Verification items for the finished model (mm, model axes). Give positions to 0.01 mm unless a question says otherwise; leave off trailing zeros. Write each loop counter-clockwise with the first axis right and the second up, starting at its lowest first coordinate (ties: lowest second). Pieces come first, ordered by that corner, then holes. Notation, with made-up numbers: (-8, -15.75) -> (1, -15.75) arc R8 ccw to (1, -1.75) -> close; hole circle Ø2 at (-15, 8.25). An arc over 180 degrees is marked (long way). Use one line per item in the form item = value. Start each with the question number.
(1) Scan lines: L1, parallel to Z at x = -72, y = 2.3; L2, parallel to Z at x = -30, y = 0.65; L3, parallel to X at y = 0.4, z = 14.5. Record each from-to range of solid material in increasing order.
(2) Section check A-A, the plane x = 60. Record the cut outline in (y, z).
(3) Section check B-B, the plane z = 0. State how many separate pieces and enclosed holes the cut face has, plus the area to 3 significant figures.
(4) Depth check by flat-ended pin: pin 1 Ø1.5 at (x, z) = (112.5, -12) entering from -Y; pin 2 Ø4 at (x, z) = (-30, 19.5) entering from -Y. Enter the tip coordinate at first touch or a pass-through.
from build123d import *

# Parameters (mm, degrees)
SKETCH1_W               = 400
SKETCH1_H               = 55
BOSS_EXTRUDE1_DEPTH     = 2.5
SKETCH2_R               = 2.5
CUT_EXTRUDE1_DEPTH      = 2.5
LPATTERN1_COUNT         = 10
LPATTERN1_PITCH         = 40
SKETCH3_R               = 7.5
CUT_EXTRUDE2_DEPTH      = 2.5
LPATTERN2_COUNT         = 4
LPATTERN2_PITCH         = 40
MIRROR1_COPY_1_SKETCH_R = 7.5
MIRROR1_COPY_1_DEPTH    = 2.5
MIRROR1_COPY_2_SKETCH_R = 7.5
MIRROR1_COPY_2_DEPTH    = 2.5
MIRROR1_COPY_3_SKETCH_R = 7.5
MIRROR1_COPY_3_DEPTH    = 2.5
FILLET1_R               = 0.5


with BuildPart() as part:
    # Sketch1 → Boss-Extrude1 (new body)
    with BuildSketch(Plane(origin=(0, 0, 0), x_dir=(1, 0, 0), z_dir=(0, 1, 0))):
        Rectangle(SKETCH1_W, SKETCH1_H)
    extrude(amount=BOSS_EXTRUDE1_DEPTH)

    # Sketch2 → Cut-Extrude1 (cut)
    with BuildSketch(Plane(origin=(0, 2.5, 0), x_dir=(1, 0, 0), z_dir=(0, 1, 0))):
        with Locations(Location((-190, 19.5, 0), (0, 0, 270))):
            Circle(SKETCH2_R)
        with Locations(Location((-170, 19.5, 0), (0, 0, 270))):
            Circle(SKETCH2_R)
        with Locations(Location((-190, -19.5, 0), (0, 0, 270))):
            Circle(SKETCH2_R)
        with Locations(Location((-170, -19.5, 0), (0, 0, 270))):
            Circle(SKETCH2_R)
    cut_extrude1 = extrude(amount=-CUT_EXTRUDE1_DEPTH, mode=Mode.SUBTRACT)

    # LPattern1: Cut-Extrude1 ×10
    with Locations(*[(i * LPATTERN1_PITCH, 0, 0) for i in range(1, LPATTERN1_COUNT)]):
        add(cut_extrude1, mode=Mode.SUBTRACT)

    # Sketch3 → Cut-Extrude2 (cut)
    with BuildSketch(Plane(origin=(0, 2.5, 0), x_dir=(1, 0, 0), z_dir=(0, 1, 0))):
        with Locations(Location((-180, 0, 0), (0, 0, 270))):
            Circle(SKETCH3_R)
    cut_extrude2 = extrude(amount=-CUT_EXTRUDE2_DEPTH, mode=Mode.SUBTRACT)

    # LPattern2: Cut-Extrude2 ×4
    with Locations(*[(i * LPATTERN2_PITCH, 0, 0) for i in range(1, LPATTERN2_COUNT)]):
        add(cut_extrude2, mode=Mode.SUBTRACT)

    # Mirror1: Cut-Extrude2 across plane
    add(cut_extrude2.mirror(Plane(origin=(0, 0, 0), x_dir=(0, 0, 1), z_dir=(1, 0, 0))), mode=Mode.SUBTRACT)

    # Mirror1 copy 1 sketch → Mirror1 copy 1 (cut)
    with BuildSketch(Plane(origin=(-40, 2.5, 0), x_dir=(-1, 0, 0), z_dir=(0, 1, 0))):
        with Locations((-180, 0)):
            Circle(MIRROR1_COPY_1_SKETCH_R)
    extrude(amount=-MIRROR1_COPY_1_DEPTH, mode=Mode.SUBTRACT)

    # Mirror1 copy 2 sketch → Mirror1 copy 2 (cut)
    with BuildSketch(Plane(origin=(-80, 2.5, 0), x_dir=(-1, 0, 0), z_dir=(0, 1, 0))):
        with Locations((-180, 0)):
            Circle(MIRROR1_COPY_2_SKETCH_R)
    extrude(amount=-MIRROR1_COPY_2_DEPTH, mode=Mode.SUBTRACT)

    # Mirror1 copy 3 sketch → Mirror1 copy 3 (cut)
    with BuildSketch(Plane(origin=(-120, 2.5, 0), x_dir=(-1, 0, 0), z_dir=(0, 1, 0))):
        with Locations((-180, 0)):
            Circle(MIRROR1_COPY_3_SKETCH_R)
    extrude(amount=-MIRROR1_COPY_3_DEPTH, mode=Mode.SUBTRACT)

    # Fillet1
    fillet1_edges = [part.edges().sort_by_distance(p)[0] for p in [
        (-200, 2.5, 0),
        (0, 2.5, 27.5),
        (200, 2.5, 0),
        (0, 0, 27.5),
        (-200, 0, 0),
        (0, 0, -27.5),
        (200, 0, 0),
        (200, 1.25, 27.5),
        (-200, 1.25, 27.5),
        (-200, 1.25, -27.5),
        (200, 1.25, -27.5),
        (0, 2.5, -27.5),
    ]]
    fillet(fillet1_edges, radius=FILLET1_R)


solid = part.part
Completed:
q1.L1 = -27.4 to -21, -18 to 18, 21 to 27.4
q1.L2 = -27.5 to -22, -17 to 17, 22 to 27.5
q1.L3 = -199.99 to 199.99
q2.outline = (0, -27) arc R0.5 ccw to (0.5, -27.5) -> (2, -27.5) arc R0.5 ccw to (2.5, -27) -> (2.5, -7.5) -> (0, -7.5) -> close; (0, 7.5) -> (2.5, 7.5) -> (2.5, 27) arc R0.5 ccw to (2, 27.5) -> (0.5, 27.5) arc R0.5 ccw to (0, 27) -> close
q3.separate_pieces = 9
q3.enclosed_holes = 0
q3.area = 700 mm²
q4.pin_1 = 0
q4.pin_2 = through
